Verification items for the finished model (mm, model axes). A direction names the side the tool comes from. Coordinates: 2 decimals unless noted, no trailing zeros. Order: outer loops, then holes, each group sorted by start corner. A loop starts at its lowest first (then second) coordinate and runs counter-clockwise, first axis right, second up.
Q1. Thickness scan on line 1 (X direction, y = -12, z = 32); line 2 (X direction, y = -4, z = -77.5). Record the ranges inside material, lowest first.
Q2. Set-up check for faces 1 (the flat face through (-12.7, -3, 61)), 2 (the flat face through (12.7, -3, 61)), 3 (the flat face through (0, 0, -5)), 4 (the flat face through (0, -3, 68.656)), 5 (the flat face through (0, -5.08, 63)): record each of +Z, -Z, +X, -X, +Y, -Y from which the full face is reachable in a straight line by a thin tool's end or side.
Q3. Depth check by flat-ended pin: P1, Ø1.5, axis at y = -8.5, z = -25.5, coming from the +X side; P2, Ø4.5, axis at x = -1, z = 61, coming from the -Y side; P3, Ø1.5, axis at y = -3.5, z = 59.5, coming from the -X side. Enter the tip coordinate at first touch or a pass-through.
Q4. Cross-section at C-C, the plane z = -107.5. Record the boundary of the cut face in (x, y), and give its area (3 significant figures).
Q5. Cross-section at B-B, the plane y = -7. Record the boundary of the cut face in (x, z), and give its area (3 significant figures).
Q6. Cross-section at A-A, the plane x = -6.5. Record the boundary of the cut face in (y, z), and give its area (3 significant figures).
Q7. Cross-section at D-D, the plane x = 9. Record the boundary of the cut face in (y, z).
from build123d import *

# Parameters (mm, degrees)
F1_DEPTH = 12.7
F0_R     = 1.4224
F2_DEPTH = 5.08


with BuildPart() as f1:
    # F0 (on Front) → F1 (new body)
    with BuildSketch(Plane.XZ):
        Polygon((0, -124.384157), (0, 53.415843), (-12.7, 53.415843), (-25.4, 53.415843), align=None)
        Polygon((12.7, 53.415843), (0, 53.415843), (0, -124.384157), (25.4, 53.415843), align=None)
    extrude(amount=F1_DEPTH)

    # F0 (on Front) → F2 (join)
    with BuildSketch(Plane.XZ):
        Polygon((-12.7, 53.415843), (0, 53.415843), (12.7, 53.415843), (12.7, 68.655843), (-12.7, 68.655843), align=None)
        with Locations((0, 61.035843)):
            Circle(F0_R, mode=Mode.SUBTRACT)
    extrude(amount=F2_DEPTH)


solid = f1.part
Check values:
1. line 1: x = -22.34 to 22.34
1. line 2: x = -6.7 to 6.7
2. face 1: +Z, -X, +Y, -Y
2. face 2: +Z, +X, +Y, -Y
2. face 3: +Z, -Z, +X, -X, +Y
2. face 4: +Z, +X, -X, +Y, -Y
2. face 5: +Z, +X, -X, -Y
3. P1: stops at x = 14.23
3. P2: stops at y = -5.08
3. P3: stops at x = -12.7
4. outline: (-2.41, -12.7) - (2.41, -12.7) - (2.41, 0) - (-2.41, 0) - close
4. area: 61.3 mm2
5. outline: (-25.4, 53.42) - (0, -124.38) - (25.4, 53.42) - close
5. area: 4,520 mm2
6. outline: (-12.7, -78.88) - (0, -78.88) - (0, 68.66) - (-5.08, 68.66) - (-5.08, 53.42) - (-12.7, 53.42) - close
6. area: 1,760 mm2
7. outline: (-12.7, -61.38) - (0, -61.38) - (0, 68.66) - (-5.08, 68.66) - (-5.08, 53.42) - (-12.7, 53.42) - close
